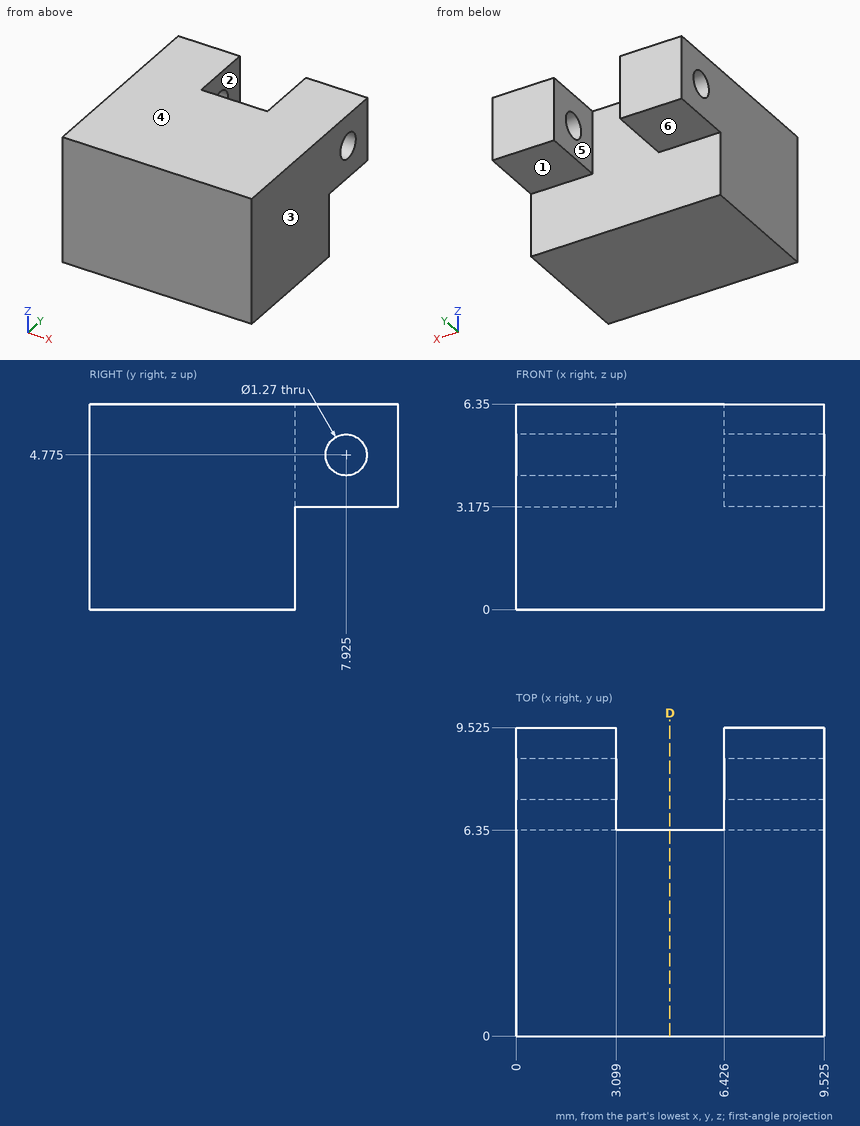
Source: three-view drawing plus pictorial views. Frame: mm from the lowest corner of the part. A direction names the side the tool comes from. Coordinates: 2 decimals unless noted, no trailing zeros. Order: outer loops, then holes, each group sorted by start corner. A loop starts at its lowest first (then second) coordinate and runs counter-clockwise, first axis right, second up. Notation, with made-up numbers: M 63.25,-6.5 L 103.25,-6.5 A31 cw 103.25,18.5 Z; hole C -10,42.25 d8. An arc over 180 degrees is marked long. Write each question's results on one line, items separated by ' | '. Start each with the question number.
1. Material intervals for L1, parallel to X at y = 9, z = 5.5 (1 decimal); L2, parallel to Y at x = 3, z = 2; L3, parallel to Z at x = 2, y = 6.5 (3 decimals), sorted ascending.
2. Draft query along X for the marked faces 1, 2 and 3. Return one class per face: +X half, -X half, draft (parallel to the pull), parting line (faces both ways), or undercut.
3. Pin query (flat end, axial travel): pin 1 (1.9 mm diameter, centred on x = 4.5, z = 2, fed in from +Y); pin 2 (1.5 mm diameter, centred on x = 8.5, y = 7.5, fed in from -Z) (3 decimals). Return the tip coordinate at first contact, or that it passes through.
4. Reachability of the marked faces 4, 5 and 6 from +Z, -Z, +X, -X, +Y, -Y: full face, straight path, thin tool, end or side. Return the list, or none.
5. Section D-D, the plane x = 4.75. Return the cut outline in (y, z).
Solution:
1) L1: 0 to 3.1, 6.4 to 9.5 | L2: 0 to 6.35 | L3: 3.175 to 6.35
2) face 1: draft | face 2: undercut | face 3: +X half
3) pin 1: y = 6.35 | pin 2: z = 3.175
4) face 4: +Z, +X, -X, +Y, -Y | face 5: +Z, -Z, +Y | face 6: -Z, +X, -X, +Y
5) outline: M 0,0 L 6.35,0 L 6.35,6.35 L 0,6.35 Z
